Autodesk Inventor part; units mm, degrees
ref_plane "YZ Plane" through (0, 0, 0) normal (1, 0, 0) x (0, 1, 0)
ref_plane "XZ Plane" through (0, 0, 0) normal (0, 1, 0) x (-1, 0, 0)
ref_plane "XY Plane" through (0, 0, 0) normal (0, 0, 1) x (1, 0, 0)
sketch "Эскиз1" plane through (0, 0, 0) normal (1, 0, 0) x (0, 1, 0)
  circle A0 centre (13.1151, 9.6132) radius 16
  line L0 (12.4181, 18.0698) -> (21.5717, 10.3101)
  line L1 (21.5717, 10.3101) -> (13.812, 1.1566)
  line L2 (13.812, 1.1566) -> (4.6584, 8.9163)
  line L3 (4.6584, 8.9163) -> (12.4181, 18.0698)
  line L4 (12.4181, 18.0698) -> (13.812, 1.1566) construction
  point P0 (0, 0)
  dimension "d0" = 32
  dimension "d2" = 12
extrude "Выдавливание1" add sketch "Эскиз1" along normal blind 10
properties part number "Задание номер 7"
Work out the finished part from the listing and answer in its coordinate system (mm). A direction names the side the tool comes from. Give positions to 0.01 mm unless a question says otherwise; leave off trailing zeros. Order: outer loops, then holes, each group sorted by start corner. A loop starts at its lowest first (then second) coordinate and runs counter-clockwise, first axis right, second up.
1. Section C-C, the plane x = 7.25 is taken. Determine the outline of the cut face in (y, z), and give its area (3 significant figures).
Result sheet:
outline: circle Ø32 at (13.12, 9.61); hole (4.66, 8.92) - (13.81, 1.16) - (21.57, 10.31) - (12.42, 18.07) - close
area: 660 mm2
2. Each of these flat-tipped pins is pushed along its axis until it touches: P1, Ø2, axis at x = 1.5, y = 5, coming from the -Z side; P2, Ø3, axis at x = 2, y = 2.5, coming from the +Z side; P3, Ø4, axis at x = 8, z = 21.5, coming from the +Y side. Where does it stop, or does it pass through?
Result sheet:
P1: stops at z = -4.72
P2: stops at z = 22.76
P3: stops at y = 25.69
3. For faces 4 (the flat face through (0, 20, 6)), 5 (the flat face through (4.93, 16.931, 14.244)), determine the directions among +Z, -Z, +X, -X, +Y, -Y from which every point of the face is accessible in a straight line to the end or side of a thin tool.
Result sheet:
face 4: +Z, -Z, -X, +Y, -Y
face 5: +X, -X
4. Section A-A, the plane y = 11.5 is taken. Determine the outline of the cut face in (x, z), and give its area (3 significant figures).
Result sheet:
outline: (0, -6.31) - (10, -6.31) - (10, 3.12) - (0, 3.12) - close; (0, 16.99) - (10, 16.99) - (10, 25.53) - (0, 25.53) - close
area: 180 mm2
5. Section B-B, the plane z = 11 is taken. Determine the outline of the cut face in (x, y).
Result sheet:
outline: (0, -2.82) - (10, -2.82) - (10, 6.42) - (0, 6.42) - close; (0, 20.76) - (10, 20.76) - (10, 29.05) - (0, 29.05) - close
6. Straight lines are drawn through the part: L1, parallel to Z at x = 4.5, y = 17; L2, parallel to Y at x = 5.5, z = 2.5; L3, parallel to Y at x = 8.5, z = 16.5. For each, find the intervals that lie inside material, in ascending order.
Result sheet:
L1: z = -5.91 to 4.92, 14.19 to 25.13
L2: y = -1.22 to 12.23, 14.95 to 27.45
L3: y = -1.33 to 11.09, 14.27 to 27.56
7. Section D-D, the plane z = 19 is taken. Determine the outline of the cut face in (x, y).
Result sheet:
outline: (0, 0.16) - (10, 0.16) - (10, 26.07) - (0, 26.07) - close
8. The mould has two halves that part along Y. Classify faces 1 (the flat face through (4.93, 9.3, 4.98)), 2 (the flat face through (10, 20, 6)), 3 (the cylindrical face through (4.93, 9.647, 25.233)): released by +Y, released by -Y, zero draft, split by the parting line, or undercut.
Result sheet:
face 1: undercut
face 2: zero draft
face 3: split by the parting line
